```python
from build123d import *

# Parameters (mm, degrees)
PAD_DEPTH    = 50
THICKNESS_T  = 1
SKETCH001_W  = 80
SKETCH001_H  = 1
PAD001_DEPTH = 50
SKETCH002_W  = 1
SKETCH002_H  = 29
PAD002_DEPTH = 50
SKETCH003_W  = 1
SKETCH003_H  = 43
PAD003_DEPTH = 50


with BuildPart() as part:
    # Sketch → Pad (new body)
    with BuildSketch(Plane.XY):
        with BuildLine():
            Line((-20, 36.5), (20, 36.5))
            ThreePointArc((40, 16.5), (34.142136, 30.642136), (20, 36.5))
            Line((40, 16.5), (40, -16.5))
            ThreePointArc((20, -36.5), (34.142136, -30.642136), (40, -16.5))
            Line((20, -36.5), (-20, -36.5))
            ThreePointArc((-40, -16.5), (-34.142136, -30.642136), (-20, -36.5))
            Line((-40, -16.5), (-40, 16.5))
            ThreePointArc((-20, 36.5), (-34.142136, 30.642136), (-40, 16.5))
        make_face()
    extrude(amount=PAD_DEPTH)

    # Thickness
    thickness_openings = [part.faces().sort_by_distance(p)[0] for p in [
        (0, 0, 50),
    ]]
    offset(amount=THICKNESS_T, openings=thickness_openings)

    # Sketch001 (on Face9 of Thickness) → Pad001 (join)
    with BuildSketch(Plane.XY):
        with Locations((0, -7)):
            Rectangle(SKETCH001_W, SKETCH001_H)
    extrude(amount=PAD001_DEPTH)

    # Sketch002 (on Face24 of Pad001) → Pad002 (join)
    with BuildSketch(Plane.XY):
        with Locations((0, -22)):
            Rectangle(SKETCH002_W, SKETCH002_H)
    extrude(amount=PAD002_DEPTH)

    # Sketch003 (on Face4 of Pad002) → Pad003 (join)
    with BuildSketch(Plane.XY):
        with Locations((0, 15)):
            Rectangle(SKETCH003_W, SKETCH003_H)
    extrude(amount=PAD003_DEPTH)


solid = part.part
```
Geometry check sheet. Reference: the model listing, model coordinates, mm. A direction names the side the tool comes from. Coordinates: 2 decimals unless noted, no trailing zeros. Loops run counter-clockwise (first coordinate to the right, second up) from the corner with the lowest first, then second, coordinate; pieces in that order, holes last. Notation, with made-up numbers: (-7, 9.25) -> (2, 9.25) arc R19 cw to (2, 43.25) -> close; hole circle Ø11 at (15, 64.5). An arc over 180 degrees is marked (long way). Put each result on its own line as item: value.
1) Cross-section at A-A on z = 35. Record the boundary of the cut face in (x, y), plus the area to 3 significant figures.
Result set:
outline: (-41, -16.5) arc R21 ccw to (-20, -37.5) -> (20, -37.5) arc R21 ccw to (41, -16.5) -> (41, 16.5) arc R21 ccw to (20, 37.5) -> (-20, 37.5) arc R21 ccw to (-41, 16.5) -> close; hole (-40, -16.5) arc R20 ccw to (-20, -36.5) -> (-0.5, -36.5) -> (-0.5, -7.5) -> (-40, -7.5) -> close; hole (-40, -6.5) -> (-0.5, -6.5) -> (-0.5, 36.5) -> (-20, 36.5) arc R20 ccw to (-40, 16.5) -> close; hole (0.5, -36.5) -> (20, -36.5) arc R20 ccw to (40, -16.5) -> (40, -7.5) -> (0.5, -7.5) -> close; hole (0.5, -6.5) -> (40, -6.5) -> (40, 16.5) arc R20 ccw to (20, 36.5) -> (0.5, 36.5) -> close
area: 427 mm^2
2) Tool access check on faces 4 (the flat face through (10, -36.5, 25)), 5 (the cylindrical face through (35.012, 31.185, 24.65)). Record the directions out of +Z, -Z, +X, -X, +Y, -Y that give a thin tool (end or side, any length) a straight path to the whole face; none if there is none.
Result set:
face 4: +Z
face 5: +Z, -Z, +X, +Y
3) Thickness scan on line 1 (X direction, y = 14, z = 17); line 2 (Y direction, x = 4, z = 2); line 3 (X direction, y = 33.5, z = 24.5). Record the ranges inside material, lowest first.
Result set:
line 1: x = -41 to -40, -0.5 to 0.5, 40 to 41
line 2: y = -37.5 to -36.5, -7.5 to -6.5, 36.5 to 37.5
line 3: x = -32.33 to -30.54, -0.5 to 0.5, 30.54 to 32.33
4) Cross-section at C-C on y = -10.5. Record the boundary of the cut face in (x, z).
Result set:
outline: (-41, 0) arc R1 ccw to (-40, -1) -> (40, -1) arc R1 ccw to (41, 0) -> (41, 50) -> (40, 50) -> (40, 0) -> (0.5, 0) -> (0.5, 50) -> (-0.5, 50) -> (-0.5, 0) -> (-40, 0) -> (-40, 50) -> (-41, 50) -> close
5) Gauge pin test, flat ends, axial feed: pin 1 Ø12 at (x, y) = (20, 23.5) entering from +Z; pin 2 Ø14.5 at (y, z) = (-27, 28.5) entering from +X; pin 3 Ø1.5 at (x, z) = (-22.5, 8) entering from +Y. Record the tip position at first contact, or that the pin passes through.
Result set:
pin 1: stops at z = 0
pin 2: stops at x = 40.75
pin 3: stops at y = 37.43
6) Release check for a two-part mould opening along X. For faces 1 (the flat face through (-20, 15, 0)), 2 (the flat face through (0, -37.5, 25)), 3 (the flat face through (-41, 0, 25)) record: released by +X, released by -X, zero draft, split by the parting line, or undercut.
Result set:
face 1: undercut
face 2: zero draft
face 3: released by -X
7) Cross-section at B-B on x = 7. Record the boundary of the cut face in (y, z), plus the area to 3 significant figures.
Result set:
outline: (-37.5, 0) arc R1 ccw to (-36.5, -1) -> (36.5, -1) arc R1 ccw to (37.5, 0) -> (37.5, 50) -> (36.5, 50) -> (36.5, 0) -> (-6.5, 0) -> (-6.5, 50) -> (-7.5, 50) -> (-7.5, 0) -> (-36.5, 0) -> (-36.5, 50) -> (-37.5, 50) -> close
area: 225 mm^2
